For this review, take the finished solid that the model builds, in its own axes (mm). A direction names the side the tool comes from. Round coordinates to 2 decimals unless told otherwise and drop trailing zeros. Loops run counter-clockwise (first coordinate to the right, second up) from the corner with the lowest first, then second, coordinate; pieces in that order, holes last.
1) Take a section at A-A (x = 6.25). State the section outline as (y, z) points (3 decimals), then the cut area to 3 significant figures.
2) Take a section at C-C (x = 0). State the section outline as (y, z) points (3 decimals), then the cut area to 3 significant figures.
3) Mouldability with a two-part tool opening along Z and no side actions: class faces 1 (the flat face through (0, 6.35, -6)), 2 (the flat face through (-7, 23, -8.89)), 3 (the cylindrical face through (-5.094, 16.099, 3.086)), 4 (the flat face through (0, 16, 9.525)) as pulls with the +Z half, pulls with the -Z half, needs draft (parallel to the pull), parting line crosses it, or undercut.
4) Take a section at B-B (z = 7.75). State the section outline as (x, y) points (3 decimals), then the cut area to 3 significant figures.
5) Insertion check: pin 1 (3 mm diameter, centred on x = -5.5, z = 7, fed in from +Y); pin 2 (3.5 mm diameter, centred on y = 16, z = 6, fed in from -X); pin 3 (2 mm diameter, centred on x = 6.92, y = 8.96, fed in from -Z). Each pin has a flat end and moves straight along its axis. Give the tip position at first contact, or say it passes through.
6) Tool access review of faces 5 (the flat face through (6, 13.589, 7)), 6 (the flat face through (-8.045, 16, 7)), 7 (the flat face through (-6, 13.589, 7)), 8 (the flat face through (6, 18.161, 7)), 9 (the flat face through (7, 23, -8.89)): name each direction out of +Z, -Z, +X, -X, +Y, -Y from which nothing blocks a thin tool from reaching the whole face with its end or side.
7) Take a section at D-D (y = 15.5). State the section outline as (x, z) points (3 decimals), then the cut area to 3 significant figures.
8) Wall thickness on L1, parallel to Z at x = 5.75, y = 23 (3 decimals); L2, parallel to Z at x = 4.75, y = 20.5 (3 decimals); L3, parallel to X at y = 15.75, z = 6.25: over which ranges is each line inside the solid? List them lowest first.
```python
from build123d import *

# Parameters (mm, degrees)
F0_R     = 5.09905
F1_DEPTH = 12.7
F3_DEPTH = 5.08
F4_W     = 19.05
F4_H     = 19.05
F5_DEPTH = 6.35
F7_DEPTH = 0.635
F8_ANGLE = -90


with BuildPart() as f1:
    # F0 (on Front) → F1 (new body)
    with BuildSketch(Plane.XZ):
        Circle(F0_R)
    extrude(amount=F1_DEPTH)

    # F2 (on face) → F3 (join)
    with BuildSketch(Plane.XZ.offset(12.7)):
        with BuildLine():
            ThreePointArc((-4.5579068554, -2.286), (-5.09905, 0), (-4.5579068554, 2.286))
            Line((-4.5579068554, 2.286), (-8.04545, 2.286))
            Line((-8.04545, 2.286), (-8.04545, -2.286))
            Line((-8.04545, -2.286), (-4.5579068554, -2.286))
        make_face()
        with BuildLine():
            Line((8.04545, 2.286), (4.5579068554, 2.286))
            ThreePointArc((4.5579068554, 2.286), (4.9619202862, 1.1745884282), (5.09905, 0))
            ThreePointArc((5.09905, 0), (4.9619202862, -1.1745884282), (4.5579068554, -2.286))
            Line((4.5579068554, -2.286), (8.04545, -2.286))
            Line((8.04545, -2.286), (8.04545, 2.286))
        make_face()
    extrude(amount=-F3_DEPTH)

    # F4 (on Front) → F5 (join)
    with BuildSketch(Plane.XZ):
        Rectangle(F4_W, F4_H)
    extrude(amount=-F5_DEPTH)

    # F6 (on face) → F7 (cut)
    with BuildSketch(Plane(origin=(0, 6.35, 0), x_dir=(-1, 0, 0), z_dir=(0, 1, 0))):
        with BuildLine():
            Line((-6.91515, 6.91515), (-5.16255, 6.91515))
            ThreePointArc((-5.16255, 6.91515), (-8.1544253447, 8.1544253447), (-6.91515, 5.16255))
            Line((-6.91515, 5.16255), (-6.91515, 6.91515))
        make_face()
        with BuildLine():
            ThreePointArc((-6.91515, 5.16255), (-5.6758746553, 5.6758746553), (-5.16255, 6.91515))
            Line((-5.16255, 6.91515), (-6.91515, 6.91515))
            Line((-6.91515, 6.91515), (-6.91515, 5.16255))
        make_face()
        with BuildLine():
            ThreePointArc((8.66775, 6.91515), (6.91515, 8.66775), (5.16255, 6.91515))
            Line((5.16255, 6.91515), (6.91515, 6.91515))
            Line((6.91515, 6.91515), (6.91515, 5.16255))
            ThreePointArc((6.91515, 5.16255), (8.1544253447, 5.6758746553), (8.66775, 6.91515))
        make_face()
        with BuildLine():
            Line((6.91515, 6.91515), (5.16255, 6.91515))
            ThreePointArc((5.16255, 6.91515), (5.6758746553, 5.6758746553), (6.91515, 5.16255))
            Line((6.91515, 5.16255), (6.91515, 6.91515))
        make_face()
        with BuildLine():
            Line((6.91515, -6.91515), (6.91515, -5.16255))
            ThreePointArc((6.91515, -5.16255), (5.6758746553, -5.6758746553), (5.16255, -6.91515))
            Line((5.16255, -6.91515), (6.91515, -6.91515))
        make_face()
        with BuildLine():
            ThreePointArc((8.66775, -6.91515), (8.1544253447, -5.6758746553), (6.91515, -5.16255))
            Line((6.91515, -5.16255), (6.91515, -6.91515))
            Line((6.91515, -6.91515), (5.16255, -6.91515))
            ThreePointArc((5.16255, -6.91515), (6.91515, -8.66775), (8.66775, -6.91515))
        make_face()
        with BuildLine():
            ThreePointArc((-5.16255, -6.91515), (-5.6758746553, -5.6758746553), (-6.91515, -5.16255))
            Line((-6.91515, -5.16255), (-6.91515, -6.91515))
            Line((-6.91515, -6.91515), (-5.16255, -6.91515))
        make_face()
        with BuildLine():
            Line((-6.91515, -6.91515), (-6.91515, -5.16255))
            ThreePointArc((-6.91515, -5.16255), (-8.1544253447, -8.1544253447), (-5.16255, -6.91515))
            Line((-5.16255, -6.91515), (-6.91515, -6.91515))
        make_face()
    extrude(amount=-F7_DEPTH, mode=Mode.SUBTRACT)


with BuildPart() as f1_1:
    # F8: moved
    add(f1.part.rotate(Axis((0, 6.35, -9.525), (1, 0, 0)), F8_ANGLE))


solid = f1_1.part
```
Response:
1. outline: (6.35, -9.525) - (7.338, -9.525) - (7.338, -8.89) - (10.581, -8.89) - (10.581, -9.525) - (21.169, -9.525) - (21.169, -8.89) - (24.412, -8.89) - (24.412, -9.525) - (25.4, -9.525) - (25.4, -3.175) - (6.35, -3.175) - close; (13.589, 4.445) - (18.161, 4.445) - (18.161, 9.525) - (13.589, 9.525) - close
1. area: 140 mm2
2. outline: (6.35, -9.525) - (25.4, -9.525) - (25.4, -3.175) - (20.974, -3.175) - (20.974, 9.525) - (10.776, 9.525) - (10.776, -3.175) - (6.35, -3.175) - close
2. area: 250 mm2
3. face 1: needs draft
3. face 2: pulls with the -Z half
3. face 3: undercut
3. face 4: pulls with the +Z half
4. outline: (-8.045, 13.589) - (-4.558, 13.589) arc R5.099 ccw to (4.558, 13.589) - (8.045, 13.589) - (8.045, 18.161) - (4.558, 18.161) arc R5.099 ccw to (-4.558, 18.161) - (-8.045, 18.161) - close
4. area: 110 mm2
5. pin 1: stops at y = 19.04
5. pin 2: stops at x = -8.05
5. pin 3: stops at z = -8.89
6. face 5: +Z, +X, -Y
6. face 6: +Z, -X, +Y, -Y
6. face 7: +Z, -X, -Y
6. face 8: +Z, +X, +Y
6. face 9: -Z
7. outline: (-9.525, -9.525) - (9.525, -9.525) - (9.525, -3.175) - (5.085, -3.175) - (5.085, 4.445) - (8.045, 4.445) - (8.045, 9.525) - (-8.045, 9.525) - (-8.045, 4.445) - (-5.085, 4.445) - (-5.085, -3.175) - (-9.525, -3.175) - close
7. area: 280 mm2
8. L1: z = -8.89 to -3.175
8. L2: z = -9.525 to -3.175
8. L3: x = -8.05 to 8.05
